Here's how the part is built. I have some questions about the finished solid (model axes, mm). A direction names the side the tool comes from. Round coordinates to 2 decimals unless told otherwise and drop trailing zeros. Loops run counter-clockwise (first coordinate to the right, second up) from the corner with the lowest first, then second, coordinate; pieces in that order, holes last. Notation, with made-up numbers: M 67.5,67 L 88.5,67 A25 ccw 88.5,80 Z; hole C 78.25,50 d8. An arc over 180 degrees is marked long. Answer as a JSON object with one key per item and string values.
from build123d import *

# Parameters (mm, degrees)
F2_DEPTH = 6.7


with BuildPart() as f2:
    # F1 (on Front) → F2 (new body)
    with BuildSketch(Plane.XZ):
        with BuildLine():
            ThreePointArc((52.5, 65), (49.5710678119, 72.0710678119), (42.5, 75))
            Line((42.5, 75), (-42.5, 75))
            ThreePointArc((-42.5, 75), (-49.5710678119, 72.0710678119), (-52.5, 65))
            Line((-52.5, 65), (-52.5, -75))
            Line((-52.5, -75), (52.5, -75))
            Line((52.5, -75), (52.5, 65))
        make_face()
        with BuildLine():
            Line((32.5, 45), (-32.5, 45))
            ThreePointArc((-32.5, 45), (-42.5, 55), (-32.5, 65))
            Line((-32.5, 65), (32.5, 65))
            ThreePointArc((32.5, 65), (42.5, 55), (32.5, 45))
        make_face(mode=Mode.SUBTRACT)
    extrude(amount=F2_DEPTH)


solid = f2.part
Item 1: On a 3-axis mill with a long thin cutter (end or side, diameter ignored), from which of +Z, -Z, +X, -X, +Y, -Y can I reach the whole of each face in a straight line? I mean faces 1 (the face through (0, -3, 65)), 2 (the face through (52.5, -3, -6)). Say none if no direction works.
Resolved:
{"face 1": "+Y, -Y", "face 2": "+Z, -Z, +X, +Y, -Y"}
Item 2: Please list where these lines run through material, in increasing order: probe 1 along Z at (x, y) = (13.5, -6); probe 2 along Z at (x, y) = (-39.5, -3.25); probe 3 along X at (y, z) = (-5.5, 61). Write a range as from..to.
Resolved:
{"probe 1": "-75..45, 65..75", "probe 2": "-75..47.86, 62.14..75", "probe 3": "-52.5..-40.5, 40.5..52.5"}
Item 3: I want a section at C-C, the plane y = -5. Please give me the cut outline in (x, z).
Resolved:
{"outline": "M -52.5,-75 L 52.5,-75 L 52.5,65 A10 ccw 42.5,75 L -42.5,75 A10 ccw -52.5,65 Z; hole M -32.5,45 L 32.5,45 A10 ccw 32.5,65 L -32.5,65 A10 ccw Z"}
Item 4: I want a section at B-B, the plane x = 11. Please give me the cut outline in (y, z), then the cut area to 3 significant figures.
Resolved:
{"outline": "M -6.7,-75 L 0,-75 L 0,45 L -6.7,45 Z; M -6.7,65 L 0,65 L 0,75 L -6.7,75 Z", "area": "871 mm²"}
Item 5: If we mould it in two halves opening along Z, with no side actions, what happens to faces 3 (the face through (42.5, -3.3, 55.2)), 4 (the face through (-52.5, -3, -4)), 5 (the face through (-1, -3, -75))? For each: pulls with the +Z half, pulls with the -Z half, needs draft (parallel to the pull), parting line crosses it, or undercut.
Resolved:
{"face 3": "undercut", "face 4": "needs draft", "face 5": "pulls with the -Z half"}
Item 6: I want a section at A-A, the plane z = 55. Please give me the cut outline in (x, y), then the cut area to 3 significant figures.
Resolved:
{"outline": "M -52.5,-6.7 L -42.5,-6.7 L -42.5,0 L -52.5,0 Z; M 42.5,-6.7 L 52.5,-6.7 L 52.5,0 L 42.5,0 Z", "area": "134 mm²"}
